from build123d import *

# Parameters (mm, degrees)
BOSS_EXTRUDE1_DEPTH     = 10
CUT_EXTRUDE2_DEPTH      = 154.297097168
FILLET1_R               = 10
FILLET2_R               = 5
CUT_EXTRUDE3_DEPTH      = 154.297097168
CUT_EXTRUDE3_DEPTH_BACK = 154.297097168
SKETCH3_W               = 7.75
SKETCH3_H               = 5.25
CUT_EXTRUDE6_DEPTH      = 154.297097168
CUT_EXTRUDE6_DEPTH_BACK = 154.297097168
SKETCH6_R               = 1.825
FILLET3_R               = 5
CUT_EXTRUDE7_DEPTH      = 154.297097168
CUT_EXTRUDE7_DEPTH_BACK = 154.297097168
SKETCH7_W               = 35.844648394
SKETCH7_H               = 9.75
SKETCH7_W_2             = 30.675
SKETCH7_H_2             = 5.25
FILLET4_R               = 2.5


# Some blends are built 0.0001 mm under size
with BuildPart() as part:
    # Sketch1 → Boss-Extrude1 (new body)
    with BuildSketch(Plane(origin=(0, 0, 0), x_dir=(0, 0, -1), z_dir=(1, 0, 0))):
        Polygon((0, 0), (150, 0), (150, 15), (75, 30), (30.773502692, 30), (25, 20), (0, 20), align=None)
    extrude(amount=-BOSS_EXTRUDE1_DEPTH)

    # Sketch2 → Cut-Extrude2 (cut, through all)
    with BuildSketch(Plane(origin=(0, 0, 0), x_dir=(0, 0, -1), z_dir=(1, 0, 0))):
        with BuildLine():
            Line((5, 11.964942747), (5, 8.035057253))
            ThreePointArc((5, 8.035057253), (10.85, 10), (5, 11.964942747))
        make_face()
    extrude(amount=-CUT_EXTRUDE2_DEPTH, mode=Mode.SUBTRACT)

    # Fillet1
    fillet1_edges = [part.edges().sort_by_distance(p)[0] for p in [
        (-5, 0, 0),
        (-5, 20, 0),
    ]]
    fillet(fillet1_edges, radius=FILLET1_R - 0.0001)  # a hair under: the kernel refuses the full size

    # Fillet2
    fillet2_edges = [part.edges().sort_by_distance(p)[0] for p in [
        (-5, 30, -30.773502692),
        (-5, 30, -75),
    ]]
    fillet(fillet2_edges, radius=FILLET2_R)

    # Sketch3 → Cut-Extrude3 (cut, two sides: drawn at the far end of the back side and taken through both)
    with BuildSketch(Plane(origin=(0, 0, 0), x_dir=(0, 0, -1), z_dir=(1, 0, 0)).offset(-CUT_EXTRUDE3_DEPTH_BACK)):
        with Locations((61.125, 7.625)):
            Rectangle(SKETCH3_W, SKETCH3_H)
        with Locations((43.875, 7.625)):
            Rectangle(SKETCH3_W, SKETCH3_H)
    extrude(amount=CUT_EXTRUDE3_DEPTH + CUT_EXTRUDE3_DEPTH_BACK, mode=Mode.SUBTRACT)

    # Sketch6 → Cut-Extrude6 (cut, two sides: drawn at the far end of the back side and taken through both)
    with BuildSketch(Plane(origin=(0, 0, 0), x_dir=(0, 0, -1), z_dir=(1, 0, 0)).offset(-CUT_EXTRUDE6_DEPTH_BACK)):
        with Locations((112.5, 7.5)):
            Circle(SKETCH6_R)
        with Locations((137.5, 7.5)):
            Circle(SKETCH6_R)
    extrude(amount=CUT_EXTRUDE6_DEPTH + CUT_EXTRUDE6_DEPTH_BACK, mode=Mode.SUBTRACT)

    # Fillet3
    fillet3_edges = [part.edges().sort_by_distance(p)[0] for p in [
        (-5, 20, -25),
    ]]
    fillet(fillet3_edges, radius=FILLET3_R)

    # Sketch7 → Cut-Extrude7 (cut, two sides: drawn at the far end of the back side and taken through both)
    with BuildSketch(Plane(origin=(0, 0, 0), x_dir=(0, 0, -1), z_dir=(1, 0, 0)).offset(-CUT_EXTRUDE7_DEPTH_BACK)):
        with Locations((51.582578235, 20.125)):
            Rectangle(SKETCH7_W, SKETCH7_H)
        with Locations((85.3375, 7.625)):
            Rectangle(SKETCH7_W_2, SKETCH7_H_2)
        Polygon((100.675, 15.25), (100.675, 19.765980486), (74.504902432, 25), (74.504902432, 15.25), align=None)
    extrude(amount=CUT_EXTRUDE7_DEPTH + CUT_EXTRUDE7_DEPTH_BACK, mode=Mode.SUBTRACT)

    # Fillet4
    # the kernel refuses this fillet: 2.5 mm, written as the material it adds along each edge
    with BuildSketch(Plane(origin=(0, 15.25, -69.504902432), x_dir=(0, 0, 1), z_dir=(-1, 0, 0)), Plane(origin=(-10, 25, -33.660254038), x_dir=(0, -1, 0), z_dir=(1, 0, 0)), Plane(origin=(0, 25, -69.504902432), x_dir=(0, -1, 0), z_dir=(-1, 0, 0)), Plane(origin=(0, 15.25, -74.504902432), x_dir=(0, 1, 0), z_dir=(-1, 0, 0)), Plane(origin=(0, 15.25, -100.675), x_dir=(0, 0, 1), z_dir=(-1, 0, 0)), Plane(origin=(0, 5, -100.675), x_dir=(0, 0, 1), z_dir=(-1, 0, 0))) as fillet4_piece_1:
        with BuildLine():
            CenterArc((FILLET4_R, FILLET4_R), FILLET4_R, 180, 90)
            Line((0, FILLET4_R), (0, 0))
            Line((0, 0), (FILLET4_R, 0))
        make_face()
    extrude(amount=10)
    with BuildSketch(Plane(origin=(-10, 15.25, -33.660254038), x_dir=(0, 1, 0), z_dir=(1, 0, 0)), Plane(origin=(-10, 5, -70), x_dir=(0, 1, 0), z_dir=(1, 0, 0)), Plane(origin=(-10, 10.25, -70), x_dir=(0, 0, -1), z_dir=(1, 0, 0)), Plane(origin=(0, 10.25, -100.675), x_dir=(0, 0, 1), z_dir=(-1, 0, 0))) as fillet4_piece_2:
        with BuildLine():
            CenterArc((FILLET4_R, -FILLET4_R), FILLET4_R, 90, 90)
            Line((0, -FILLET4_R), (0, 0))
            Line((0, 0), (FILLET4_R, 0))
        make_face()
    extrude(amount=10)
    with BuildSketch(Plane(origin=(-10, 25, -74.504902432), x_dir=(0, -0.1961161351381845, -0.9805806756909201), z_dir=(1, 0, 0))) as fillet4_piece_3:
        with BuildLine():
            CenterArc((FILLET4_R * 1.21980390272, -FILLET4_R), FILLET4_R, 90, 101.309932474)
            Line((FILLET4_R * 0.239223227028, -FILLET4_R * 1.19611613514), (0, 0))
            Line((0, 0), (FILLET4_R * 1.21980390272, 0))
        make_face()
    extrude(amount=10)
    with BuildSketch(Plane(origin=(-10, 19.765980486, -100.675), x_dir=(0, 0.19611613513818169, 0.9805806756909206), z_dir=(1, 0, 0))) as fillet4_piece_4:
        with BuildLine():
            CenterArc((FILLET4_R * 0.819803902719, FILLET4_R), FILLET4_R, 191.309932474, 78.690067526)
            Line((-FILLET4_R * 0.160776772972, FILLET4_R * 0.803883864862), (0, 0))
            Line((0, 0), (FILLET4_R * 0.819803902719, 0))
        make_face()
    extrude(amount=10)


solid = part.part
Here's how the part is built. I have some questions about the finished solid (model axes, mm). A direction names the side the tool comes from. Round coordinates to 2 decimals unless told otherwise and drop trailing zeros. Write each loop counter-clockwise with the first axis right and the second up, starting at its lowest first coordinate (ties: lowest second). Pieces come first, ordered by that corner, then holes.
1. I need wall thicknesses on L1, parallel to Y at x = -9, z = -40.5; L2, parallel to Y at x = -0.75, z = -84; L3, parallel to Y at x = -4, z = -36. Which ranges of each line are inside material? Lowest first, please.
2. Will these pins go through, and if not, where does the flat tip stop? pin 1 Ø5 at (x, z) = (-5.5, -89) entering from +Y; pin 2 Ø1.5 at (x, z) = (-2, -120.5) entering from +Y; pin 3 Ø4 at (x, y) = (-6, 21) entering from +Z.
3. For faces 4 (the flat face through (-5, 8, -40)), 5 (the cylindrical face through (-5.07, 29.348, -31.192)), which set-ups out of +Z, -Z, +X, -X, +Y, -Y let a thin tool reach every point of the face, with its end or its side?
4. Suppose I cut it at D-D (y = 16.5). List the corners of the cut face in (x, z) for me.
5. Suppose I cut it at B-B (z = -137.5). List the corners of the cut face in (x, y) for me (3 decimals).
6. Suppose I cut it at A-A (z = -112.5). List the corners of the cut face in (x, y) for me (3 decimals).
7. Suppose I cut it at C-C (x = -8.75). State how many separate pieces and enclosed holes the cut face has, and give its area (3 significant figures).
8. If we mould it in two halves opening along Z, with no side actions, what happens to faces 1 (the cylindrical face through (-5.07, 20.688, -24.645)), 2 (the flat face through (-10, 13, -78)), 3 (the flat face through (-5, 10.25, -85))? For each: released by +Z, released by -Z, zero draft, split by the parting line, or undercut.
Answer sheet:
1. L1: y = 0 to 5, 10.25 to 15.25, 25 to 30
1. L2: y = 0 to 5, 10.25 to 15.25, 23.1 to 28.2
1. L3: y = 0 to 15.26, 24.99 to 30
2. pin 1: stops at y = 27.7
2. pin 2: stops at y = 21.05
2. pin 3: stops at z = -5.64
3. face 4: +X, -X
3. face 5: +Z, +X, -X, +Y
4. outline: (-10, -142.5) - (0, -142.5) - (0, -100.34) - (-10, -100.34) - close; (-10, -74.84) - (0, -74.84) - (0, -69.17) - (-10, -69.17) - close; (-10, -34) - (0, -34) - (0, -2.4) - (-10, -2.4) - close
5. outline: (-10, 0) - (0, 0) - (0, 5.675) - (-10, 5.675) - close; (-10, 9.325) - (0, 9.325) - (0, 17.5) - (-10, 17.5) - close
6. outline: (-10, 0) - (0, 0) - (0, 5.675) - (-10, 5.675) - close; (-10, 9.325) - (0, 9.325) - (0, 22.5) - (-10, 22.5) - close
7. separate pieces: 1
7. enclosed holes: 8
7. area: 2,800 mm2
8. face 1: released by +Z
8. face 2: zero draft
8. face 3: undercut
